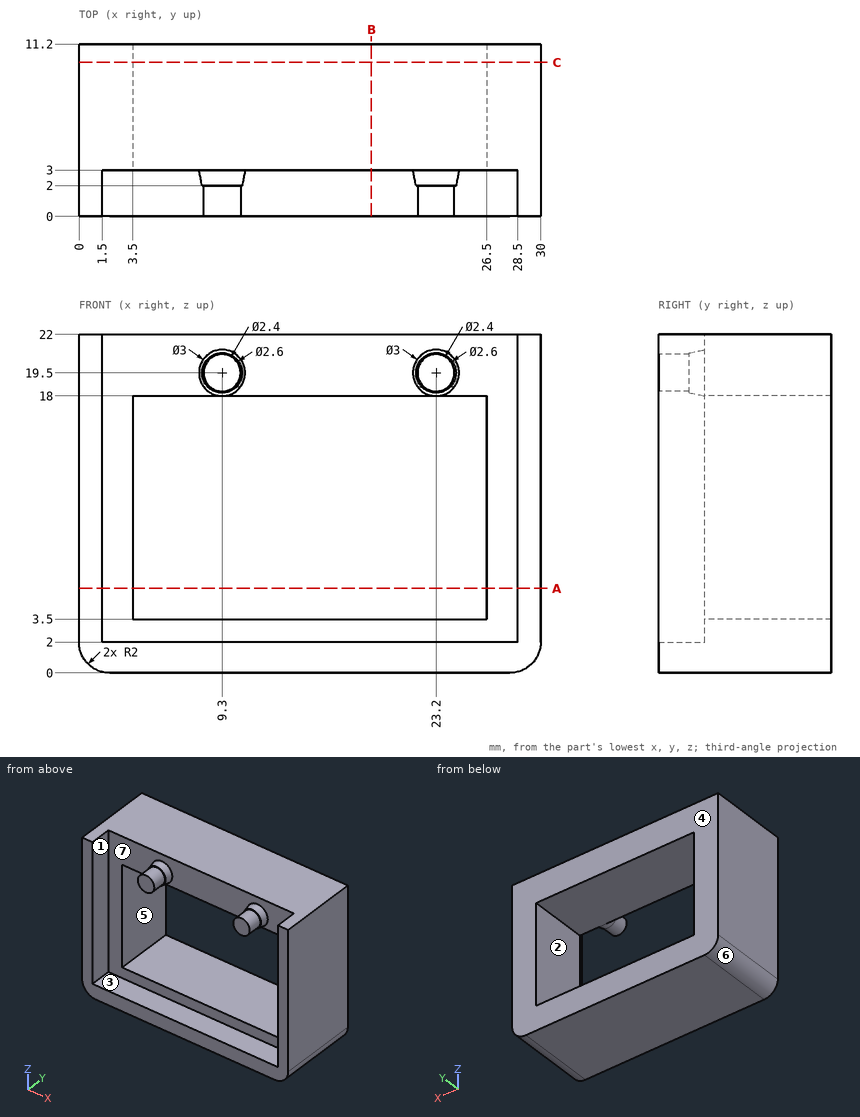
Here's the drawing with two shaded views (mm, measured from the low corner). I have some questions. A direction names the side the tool comes from. Give positions to 0.01 mm unless a question says otherwise; leave off trailing zeros. Loops run counter-clockwise (first coordinate to the right, second up) from the corner with the lowest first, then second, coordinate; pieces in that order, holes last. Notation, with made-up numbers: (-24.75, -3) - (0.25, -3) arc R18 cw to (0.25, 30) - close; hole circle Ø9 at (86, 85.25). An arc over 180 degrees is marked (long way). One line per item, written item: value.
(1) I'm going to push flat-ended pins straight in: pin 1 (5 mm diameter, centred on x = 5, y = 6, fed in from -Z); pin 2 (3.5 mm diameter, centred on x = 17.5, y = 1, fed in from +Z); pin 3 (5 mm diameter, centred on x = 16.5, z = 19, fed in from -Y). Where does each tip first touch, or does it pass through?
Verdict:
pin 1: z = 0
pin 2: z = 2
pin 3: y = 3
(2) If we section it at C-C, the plane y = 10: List the corners of the cut face in (x, z) for me.
Verdict:
outline: (0, 2) arc R2 ccw to (2, 0) - (28, 0) arc R2 ccw to (30, 2) - (30, 22) - (0, 22) - close; hole (3.5, 3.5) - (26.5, 3.5) - (26.5, 18) - (3.5, 18) - close
(3) If we section it at A-A, the plane z = 5.5: List the corners of the cut face in (x, y) for me, plus the area to 3 significant figures.
Verdict:
outline: (0, 0) - (1.5, 0) - (1.5, 3) - (3.5, 3) - (3.5, 11.2) - (0, 11.2) - close; (26.5, 3) - (28.5, 3) - (28.5, 0) - (30, 0) - (30, 11.2) - (26.5, 11.2) - close
area: 66.4 mm^2
(4) On a 3-axis mill with a long thin cutter (end or side, diameter ignored), from which of +Z, -Z, +X, -X, +Y, -Y can I reach the whole of each face in a straight line? I mean the marked faces 1, 2 and 3. Say none if no direction works.
Verdict:
face 1: +Z, -Y
face 2: +Y, -Y
face 3: -Y
(5) If we section it at B-B, the plane x = 19: List the corners of the cut face in (y, z) for me.
Verdict:
outline: (0, 0) - (11.2, 0) - (11.2, 3.5) - (3, 3.5) - (3, 2) - (0, 2) - close; (3, 18) - (11.2, 18) - (11.2, 22) - (3, 22) - close
(6) I need wall thicknesses on line 1 along Z through (x, y) = (15.5, 8); line 2 along X through (y, z) = (1, 11.5); line 3 along X through (y, z) = (8, 10.5). Which ranges of each line are inside material? Lowest first, please.
Verdict:
line 1: 0 to 3.5, 18 to 22
line 2: 0 to 1.5, 28.5 to 30
line 3: 0 to 3.5, 26.5 to 30
(7) If we mould it in two halves opening along X, with no side actions, what happens to the marked faces 4, 5, 6 and 7? For each: released by +X, released by -X, zero draft, split by the parting line, or undercut.
Verdict:
face 4: zero draft
face 5: undercut
face 6: released by -X
face 7: undercut
